Build history of the part. All positions in model axes, mm. Round coordinates to 2 decimals unless told otherwise and drop trailing zeros. Write each loop counter-clockwise with the first axis right and the second up, starting at its lowest first coordinate (ties: lowest second). Pieces come first, ordered by that corner, then holes. Notation, with made-up numbers: M 7.25,-6.5 L 23.25,-6.5 A23 cw 23.25,23.5 Z; hole C -15,13 d5. An arc over 180 degrees is marked long. Write item = value, one per line.
Autodesk Inventor part; units mm, degrees
ref_plane "YZ Plane" through (0, 0, 0) normal (1, 0, 0) x (0, 1, 0)
ref_plane "XZ Plane" through (0, 0, 0) normal (0, 1, 0) x (-1, 0, 0)
ref_plane "XY Plane" through (0, 0, 0) normal (0, 0, 1) x (1, 0, 0)
sketch "Sketch1" plane through (0, 0, 0) normal (0, 0, 1) x (1, 0, 0)
  line L0 (0, 0) -> (12.7, 0)
  line L1 (12.7, 0) -> (12.7, 50.8)
  line L2 (12.7, 50.8) -> (0, 50.8)
  line L3 (0, 50.8) -> (0, 0)
  dimension "d0" = 12.7
  dimension "d1" = 50.8
extrude "Extrusion1" add sketch "Sketch1" along normal blind 12.7
sketch "Sketch5" plane through (0, 0, 12.7) normal (0, 0, 1) x (1, 0, 0)
  line L0 (12.7, 0) -> (12.7, 50.8)
  line L1 (12.7, 50.8) -> (0, 50.8)
  line L2 (0, 0) -> (12.7, 0)
  point P0 (6.35, 38.1)
  point P1 (6.35, 12.7)
  point P2 (6.35, 50.8)
  dimension "d19" = 6.35
  dimension "d20" = 12.7
  dimension "d21" = 6.35
  dimension "d22" = 12.7
hole "Hole1" at (6.35, 38.1, 12.7) at (6.35, 12.7, 12.7) direction (0, 0, -1) diameter 4.5 end through all
sketch "Sketch6" plane through (0, 0, 12.7) normal (0, 0, 1) x (1, 0, 0)
  line L0 (12.7, 50.8) -> (0, 50.8)
  line L1 (0, 50.8) -> (0, 45.8)
  line L2 (0, 50.8) -> (0, 0)
  line L3 (12.7, 0) -> (12.7, 50.8)
  line L4 (12.7, 45.8) -> (12.7, 50.8)
  line L5 (12.7, 50.8) -> (0, 50.8)
  line L6 (0, 45.8) -> (12.7, 45.8)
  dimension "d32" = 5
extrude "Extrusion4" cut sketch "Sketch6" against normal blind 12.7
sketch "Sketch7" plane through (0, 0, 12.7) normal (0, 0, 1) x (1, 0, 0)
  line L0 (0, 45.8) -> (0, 0)
  line L1 (0, 0) -> (0, 5)
  line L2 (12.7, 0) -> (12.7, 45.8)
  line L3 (12.7, 5) -> (12.7, 0)
  line L4 (0, 0) -> (12.7, 0)
  line L5 (12.7, 0) -> (0, 0)
  line L6 (0, 5) -> (12.7, 5)
  dimension "d35" = 5
extrude "Extrusion5" cut sketch "Sketch7" against normal blind 12.7
fillet "Fillet3" radius 6 2 edges at (12.7, 45.8, 6.35) (0, 45.8, 6.35)
fillet "Fillet4" radius 6 2 edges at (12.7, 5, 6.35) (0, 5, 6.35)
sketch "Sketch8" plane through (12.7, 39.8, 12.7) normal (1, 0, 0) x (0, 0, -1)
  circle A0 centre (6.35, -12.044) radius 2.25
  line L0 (12.7, -28.8) -> (12.7, 0)
  line L1 (12.7, -28.8) -> (0, -28.8)
  line L2 (0, -34.8) -> (12.7, -34.8)
  point P0 (12.7, -39.8)
  dimension "d43" = 6.35
  dimension "d44" = 4.5
  dimension "d49" = 16.756
extrude "Extrusion6" cut sketch "Sketch8" against normal blind 12.7
properties part number "Slider7"
1. Band-saw the part on D-D (x = 9.25). List the corners of the cut face in (y, z).
Responses:
outline = M 5.57,0 L 45.23,0 L 45.23,12.7 L 5.57,12.7 Z; hole C 27.76,6.35 d4.5
2. Band-saw the part on B-B (y = 38.1). List the corners of the cut face in (x, z).
Responses:
outline = M 0,0 L 4.1,0 L 4.1,12.7 L 0,12.7 Z; M 8.6,0 L 12.7,0 L 12.7,12.7 L 8.6,12.7 Z
3. Mould opens along Z. For faces 1 (the face through (0, 26, 8)), 2 (the face through (6, 26, 0)), 3 (the face through (6, 26, 12.7)), 4 (the face through (6.439, 29.653, 5.14)) say: pulls with the +Z half, pulls with the -Z half, needs draft (parallel to the pull), parting line crosses it, or undercut.
Responses:
face_1 = needs draft
face_2 = pulls with the -Z half
face_3 = pulls with the +Z half
face_4 = undercut
4. Band-saw the part on C-C (z = 2.75). List the corners of the cut face in (x, y), plus the area to 3 significant figures.
Responses:
outline = M 0,11 A6 ccw 6,5 L 6.7,5 A6 ccw 12.7,11 L 12.7,39.8 A6 ccw 6.7,45.8 L 6,45.8 A6 ccw 0,39.8 Z; hole C 6.35,12.7 d4.5; hole C 6.35,38.1 d4.5
area = 455 mm²
5. Probe probe 1 along Y at (x, z) = (6.35, 6.25); probe 2 along Y at (x, z) = (6.35, 3.25); probe 3 along Y at (x, z) = (7.75, 9.5). List the from-to ranges inside material, lowest first.
Responses:
probe_1 = 5 to 10.45, 14.95 to 25.51, 30 to 35.85, 40.35 to 45.8
probe_2 = 5 to 10.45, 14.95 to 35.85, 40.35 to 45.8
probe_3 = 5.09 to 10.94, 14.46 to 36.34, 39.86 to 45.71
6. Band-saw the part on A-A (z = 6.35). List the corners of the cut face in (x, y).
Responses:
outline = M 0,11 A6 ccw 6,5 L 6.7,5 A6 ccw 12.7,11 L 12.7,25.51 L 0,25.51 Z; M 0,30.01 L 12.7,30.01 L 12.7,39.8 A6 ccw 6.7,45.8 L 6,45.8 A6 ccw 0,39.8 Z; hole C 6.35,12.7 d4.5; hole C 6.35,38.1 d4.5
7. Flat gauge pins, fed straight in: pin 1 (2 mm diameter, centred on x = 11, z = 6, fed in from +Y); pin 2 (2 mm diameter, centred on x = 8, z = 4.5, fed in from -Y). Where does each tip first touch, or does it go through?
Responses:
pin_1 = 44.81
pin_2 = 5.01
